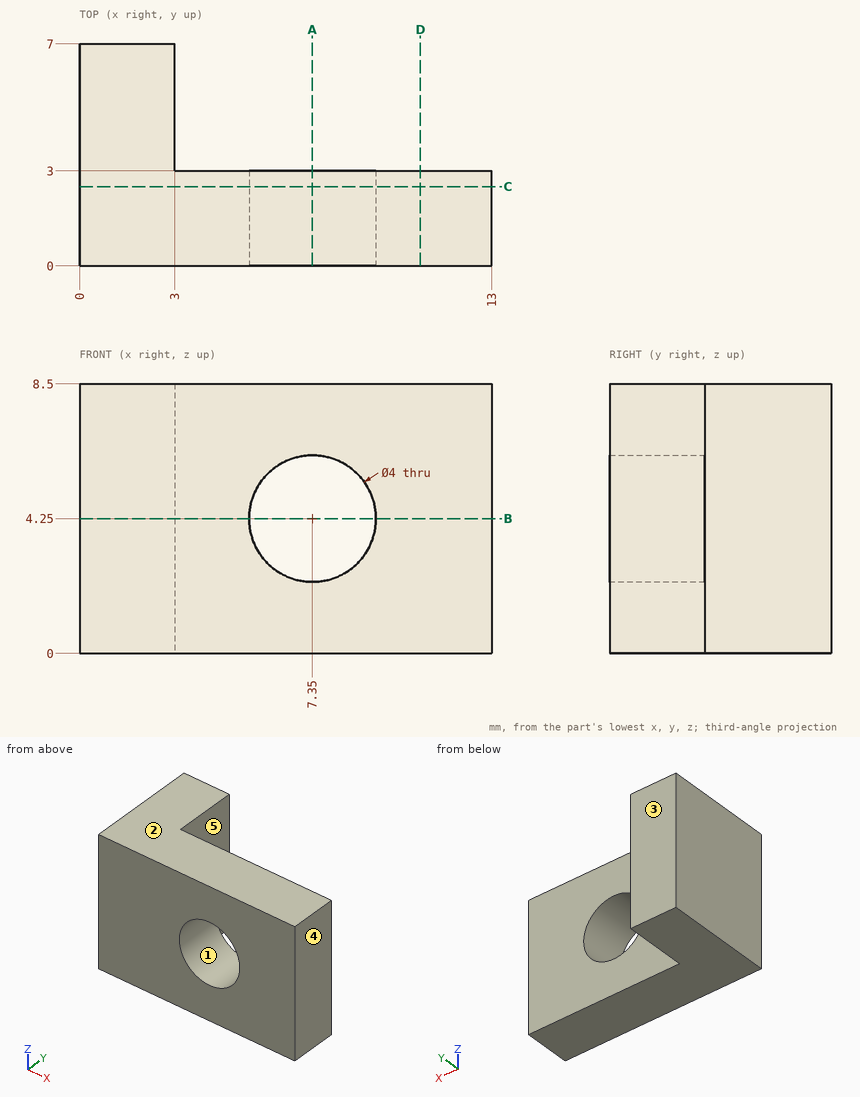
For this review, use the dimensioned drawing (mm, ordinates from the lowest corner) and the shaded views. A direction names the side the tool comes from. Round coordinates to 2 decimals unless told otherwise and drop trailing zeros. Write each loop counter-clockwise with the first axis right and the second up, starting at its lowest first coordinate (ties: lowest second). Pieces come first, ordered by that corner, then holes. Notation, with made-up numbers: M 43,-26 L 52,-26 A21 ccw 52,-16 Z; hole C -1,54.25 d10. An arc over 180 degrees is marked long. Answer as CSV lines item,"result". Start each with the question number.
Q1. Wall thickness on line 1 along Z through (x, y) = (7.35, 0.75); line 2 along X through (y, z) = (2.2, 4.25); line 3 along X through (y, z) = (3.75, 5): over which ranges is each line inside the solid? List them lowest first.
Q2. Consider section C-C, the plane y = 2.5. Give the boundary of the cut face in (x, z), then the cut area to 3 significant figures.
Q3. The part is to be moulded in two halves that separate along Z. For the marked faces 1, 2 and 3, say which applies: +Z half, -Z half, draft (parallel to the pull), parting line (faces both ways), or undercut.
Q4. Consider section D-D, the plane x = 10.75. Give the boundary of the cut face in (y, z), then the cut area to 3 significant figures.
Q5. Tool access review of the marked faces 4 and 5: name each direction out of +Z, -Z, +X, -X, +Y, -Y from which nothing blocks a thin tool from reaching the whole face with its end or side.
Q6. Consider section A-A, the plane x = 7.35. Give the boundary of the cut face in (y, z).
Q7. Clearance check with flat-ended pins moving along their axes: P1, Ø2, axis at x = 2.5, y = 2.5, coming from the -Z side; P2, Ø1.2, axis at y = 4.5, z = 3, coming from the +X side. State where each tip first meets the part, or that it passes through.
Q8. Consider section B-B, the plane z = 4.25. Give the boundary of the cut face in (x, y).
Result set:
1,line 1,"z = 0 to 2.25, 6.25 to 8.5"
1,line 2,"x = 0 to 5.35, 9.35 to 13"
1,line 3,"x = 0 to 3"
2,outline,"M 0,0 L 13,0 L 13,8.5 L 0,8.5 Z; hole C 7.35,4.25 d4"
2,area,"97.9 mm²"
3,face 1,"undercut"
3,face 2,"+Z half"
3,face 3,"draft"
4,outline,"M 0,0 L 3,0 L 3,8.5 L 0,8.5 Z"
4,area,"25.5 mm²"
5,face 4,"+Z, -Z, +X, +Y, -Y"
5,face 5,"+Z, -Z, +X, +Y"
6,outline,"M 0,0 L 3,0 L 3,2.25 L 0,2.25 Z; M 0,6.25 L 3,6.25 L 3,8.5 L 0,8.5 Z"
7,P1,"stops at z = 0"
7,P2,"stops at x = 3"
8,outline,"M 0,0 L 5.35,0 L 5.35,3 L 3,3 L 3,7 L 0,7 Z; M 9.35,0 L 13,0 L 13,3 L 9.35,3 Z"
